The figure shows three views and two pictorial views of one solid part (mm, origin at its lowest corner). Answer the questions. Round coordinates to 2 decimals unless told otherwise and drop trailing zeros. Write each loop counter-clockwise with the first axis right and the second up, starting at its lowest first coordinate (ties: lowest second). Pieces come first, ordered by that corner, then holes. Notation, with made-up numbers: M 1.5,38.25 L 19.5,38.25 A14 cw 19.5,59.25 Z; hole C 57,48.5 d7. An arc over 180 degrees is marked long. Use one line per item in the form item = value. Start each with the question number.
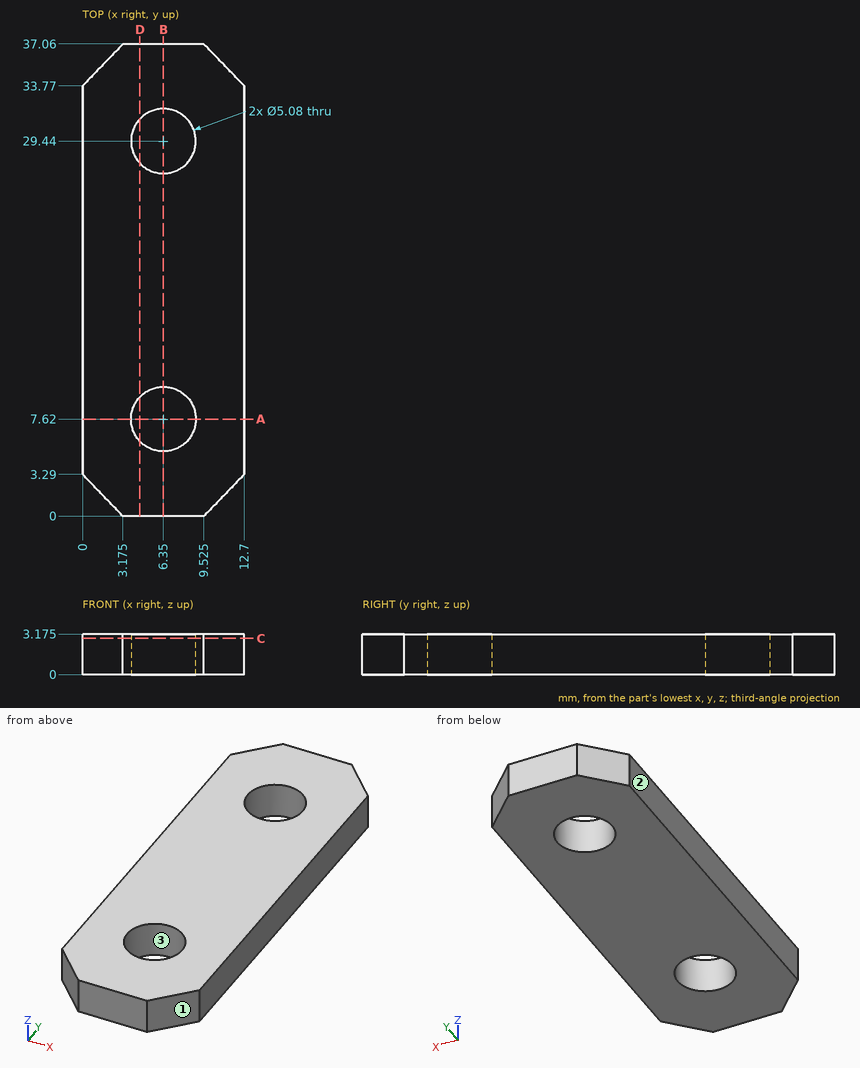
Q1. Find section C-C on z = 2.85. Count the separate pieces of the cut face and the enclosed holes in it, and give its area (3 significant figures).
Q2. Straight lines are drawn through the part: line 1 (Y direction, x = 6.35, z = 2.3); line 2 (X direction, y = 7.62, z = 1.8); line 3 (Y direction, x = 8, z = 3). For each, find the intervals that lie inside material, in ascending order. Write a range as [from, to].
Q3. For a pull along X with two mould halves and no side action, classify the marked faces 1, 2 and 3 as +X half, -X half, draft (parallel to the pull), parting line (faces both ways), or undercut.
Q4. Find section B-B on x = 6.35. Write down the section's boundary in (y, z) (1 decimal).
Q5. Find section D-D on x = 4.5. Write down the section's boundary in (y, z) (1 decimal).
Q6. Find section A-A on y = 7.62. Write down the section's boundary in (x, z) (1 decimal), and give its area (3 significant figures).
Response:
q1.separate_pieces = 1
q1.enclosed_holes = 2
q1.area = 409 mm²
q2.line_1 = [0, 5.08], [10.16, 26.9], [31.98, 37.06]
q2.line_2 = [0, 3.81], [8.89, 12.7]
q2.line_3 = [0, 5.69], [9.55, 27.51], [31.37, 37.06]
q3.face_1 = +X half
q3.face_2 = -X half
q3.face_3 = undercut
q4.outline = M 0,0 L 5.1,0 L 5.1,3.2 L 0,3.2 Z; M 10.2,0 L 26.9,0 L 26.9,3.2 L 10.2,3.2 Z; M 32,0 L 37.1,0 L 37.1,3.2 L 32,3.2 Z
q5.outline = M 0,0 L 5.9,0 L 5.9,3.2 L 0,3.2 Z; M 9.4,0 L 27.7,0 L 27.7,3.2 L 9.4,3.2 Z; M 31.2,0 L 37.1,0 L 37.1,3.2 L 31.2,3.2 Z
q6.outline = M 0,0 L 3.8,0 L 3.8,3.2 L 0,3.2 Z; M 8.9,0 L 12.7,0 L 12.7,3.2 L 8.9,3.2 Z
q6.area = 24.2 mm²
